Check sheet for the modelled part. Datum: model origin and axes. Units: mm. Face numbers are marked on the shaded views. A direction names the side the tool comes from. Coordinates: 2 decimals unless noted, no trailing zeros. Order: outer loops, then holes, each group sorted by start corner. A loop starts at its lowest first (then second) coordinate and runs counter-clockwise, first axis right, second up. Notation, with made-up numbers: (73.25, 26) -> (110.25, 26) arc R8 ccw to (110.25, 37) -> close; hole circle Ø2 at (88, -24.5). An arc over 180 degrees is marked (long way). Put each result on its own line as item: value. Start each with the question number.
```python
from build123d import *

# Parameters (mm, degrees)
CYLINDER008_R     = 2
CYLINDER008_DEPTH = 3.2
CYLINDER009_R     = 1.7
CYLINDER009_DEPTH = 30
CYLINDER007_R     = 37.75
CYLINDER007_DEPTH = 63
CYLINDER013_R     = 42.75
CYLINDER013_DEPTH = 45
CYLINDER012_R     = 49.75
CYLINDER012_DEPTH = 32.5
SKETCH009_R       = 2.2
POCKET008_DEPTH   = 5
POCKET010_DEPTH   = 25
PAD002_DEPTH      = 5
SKETCH018_W       = 2.5
SKETCH018_H       = 5
POCKET016_DEPTH   = 27.501
SKETCH020_R       = 4
POCKET018_DEPTH   = 5
SKETCH021_R       = 4.4
POCKET019_DEPTH   = 2.5
SKETCH022_R       = 7
POCKET020_DEPTH   = 5
SKETCH023_R       = 1.7
POCKET021_DEPTH   = 5
PAD010_DEPTH      = 15


with BuildPart() as cylinder008:
    # Cylinder008 → Cylinder008 (new body)
    with BuildSketch(Plane.XY.offset(64.8)):
        Circle(CYLINDER008_R)
    extrude(amount=CYLINDER008_DEPTH)


with BuildPart() as fusion005:
    # Cylinder009 → Cylinder009 (new body)
    with BuildSketch(Plane.XY.offset(63)):
        Circle(CYLINDER009_R)
    extrude(amount=CYLINDER009_DEPTH)

    # Fusion005: union Cylinder008
    add(cylinder008.part)


with BuildPart() as cylinder007:
    # Cylinder007 → Cylinder007 (new body)
    with BuildSketch(Plane.XY):
        Circle(CYLINDER007_R)
    extrude(amount=CYLINDER007_DEPTH)


with BuildPart() as fusion006:
    # Cylinder013 → Cylinder013 (new body)
    with BuildSketch(Plane.XY):
        Circle(CYLINDER013_R)
    extrude(amount=CYLINDER013_DEPTH)

    # Fusion006: union Cylinder007
    add(cylinder007.part)


with BuildPart() as obj1:
    # Cylinder012 → Cylinder012 (new body)
    with BuildSketch(Plane.XY.offset(35.5)):
        Circle(CYLINDER012_R)
    extrude(amount=CYLINDER012_DEPTH)

    # Cut008: cut Fusion006
    add(fusion006.part, mode=Mode.SUBTRACT)

    # Cut009: cut Fusion005
    add(fusion005.part, mode=Mode.SUBTRACT)

    # Sketch009 (on Face3 of Cut009) → Pocket008 (cut)
    with BuildSketch(Plane.XY.offset(68)):
        with Locations((0, 28)):
            Circle(SKETCH009_R)
        with Locations((28, 0)):
            Circle(SKETCH009_R)
        with Locations((0, -33)):
            Circle(SKETCH009_R)
        with Locations((-28, 0)):
            Circle(SKETCH009_R)
    extrude(amount=-POCKET008_DEPTH, mode=Mode.SUBTRACT)

    # Sketch011 → Pocket010 (cut)
    with BuildSketch(Plane(origin=(0, 60, -1), x_dir=(1, 0, 0), z_dir=(0, -1, 0))):
        with BuildLine():
            ThreePointArc((3.4, 59.599979), (1.2e-05, 63), (-3.4, 59.600003))
            Line((-3.4, 59.600003), (-3.4, 0))
            Line((-3.4, 0), (3.4, 0))
            Line((3.4, 59.599979), (3.4, 0))
        make_face()
    extrude(amount=POCKET010_DEPTH, mode=Mode.SUBTRACT)

    # Sketch017 (on Face2 of Pocket010) → Pad002 (join)
    with BuildSketch(Plane(origin=(0, 0, 35.5), x_dir=(1, 0, 0), z_dir=(0, 0, -1))):
        with BuildLine():
            ThreePointArc((20.231067, 45.395694), (-0.005277, 49.699749), (-20.240706, 45.391396))
            Line((-7.40759, 82.752427), (-20.240706, 45.391396))
            ThreePointArc((7.358623, 82.756756), (-0.025675, 86.818946), (-7.40759, 82.752427))
            Line((7.358623, 82.756756), (20.231067, 45.395694))
        make_face()
    extrude(amount=-PAD002_DEPTH)

    # Sketch018 (on Face22 of Pad002) → Pocket016 (cut, through all)
    with BuildSketch(Plane(origin=(0, 0, 63), x_dir=(1, 0, 0), z_dir=(0, 0, -1))):
        with Locations((0, 67.5)):
            Rectangle(SKETCH018_W, SKETCH018_H)
    extrude(amount=POCKET016_DEPTH, mode=Mode.SUBTRACT)

    # Sketch020 → Pocket018 (cut)
    with BuildSketch(Plane.XY.offset(68)):
        Circle(SKETCH020_R)
    extrude(amount=-POCKET018_DEPTH, mode=Mode.SUBTRACT)

    # Sketch021 (on Face26 of Pocket018) → Pocket019 (cut)
    with BuildSketch(Plane(origin=(0, 0, 63), x_dir=(1, 0, 0), z_dir=(0, 0, -1))):
        with Locations((0, 33)):
            Circle(SKETCH021_R)
        with Locations((28, 0)):
            Circle(SKETCH021_R)
        with Locations((-28, 0)):
            Circle(SKETCH021_R)
        with Locations((0, -28)):
            Circle(SKETCH021_R)
    extrude(amount=-POCKET019_DEPTH, mode=Mode.SUBTRACT)

    # Sketch022 (on Face2 of Pocket019) → Pocket020 (cut)
    with BuildSketch(Plane.XY.offset(68)):
        Circle(SKETCH022_R)
    extrude(amount=-POCKET020_DEPTH, mode=Mode.SUBTRACT)

    # Sketch023 (on Face2 of Pocket020) → Pocket021 (cut)
    with BuildSketch(Plane.XY.offset(68)):
        with Locations((-15.5, -7)):
            Circle(SKETCH023_R)
        with Locations((15.5, -7)):
            Circle(SKETCH023_R)
        with Locations((-7.75, -20.4)):
            Circle(SKETCH023_R)
        with Locations((7.75, -20.4)):
            Circle(SKETCH023_R)
        with Locations((-7.75, 6.45)):
            Circle(SKETCH023_R)
        with Locations((7.75, 6.45)):
            Circle(SKETCH023_R)
    extrude(amount=-POCKET021_DEPTH, mode=Mode.SUBTRACT)

    # Sketch051 → Pad010 (join)
    with BuildSketch(Plane(origin=(0, 0, 35.5), x_dir=(1, 0, 0), z_dir=(0, 0, -1))):
        with BuildLine():
            Line((3.4, -42), (3.4, -47))
            ThreePointArc((3.4, -47), (0, 47.122818), (-3.4, -47))
            Line((-3.4, -47), (-3.4, -42))
            ThreePointArc((3.4, -42), (0, 42.137394), (-3.4, -42))
        make_face()
    extrude(amount=-PAD010_DEPTH)


with BuildPart() as obj1_1:
    # Body001 placement: moved
    add(obj1.part.moved(Location((0, 0, -68))))


solid = obj1_1.part
```
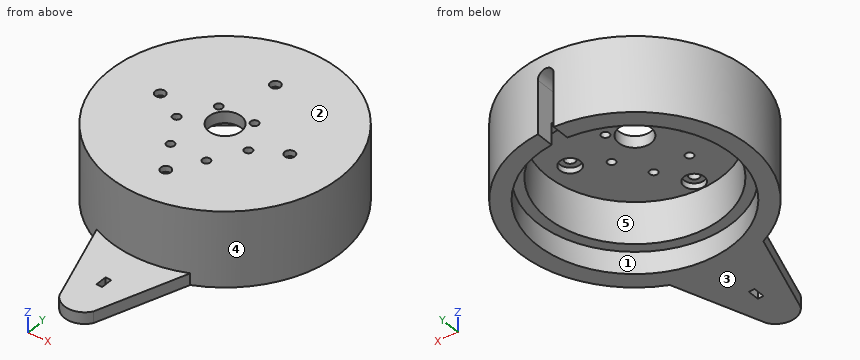
1) Sectioned sample at C-C (x = 15.5). Record the boundary of the cut face in (y, z), plus the area to 3 significant figures.
2) Gauge pin test, flat ends, axial feed: pin 1 (4 mm diameter, centred on x = 7.75, y = -20.4, fed in from -Z); pin 2 (1.5 mm diameter, centred on y = -19.5, z = -6.5, fed in from -X); pin 3 (5 mm diameter, centred on x = 24, z = -18.5, fed in from +Y); pin 4 (7 mm diameter, centred on x = 0, y = 28, fed in from +Z). Record the tip position at first contact, or that the pin passes through.
3) Sectioned sample at D-D (y = -33). Record the boundary of the cut face in (x, z).
4) Sectioned sample at A-A (z = -29.5). Record the boundary of the cut face in (x, y), plus the area to 3 significant figures.
5) Scan lines: line 1 along Y through (x, z) = (0, -1); line 2 along Y through (x, z) = (7.75, -1.1); line 3 along Y through (x, z) = (0, -4). Record each from-to range of solid material in increasing order. Write a range as [from, to].
6) Mould release check, pull along Y, two halves, no side actions. Record for the marked faces 3, 4 and 5: +Y half, -Y half, draft (parallel to the pull), parting line (faces both ways), or undercut.
7) Access from +Z, -Z, +X, -X, +Y, -Y to the whole of each face (thin tool, end or side, straight path). Record for the marked faces 1 and 2.
8) Sectioned sample at B-B (y = 0). State how many separate pieces and enclosed holes the cut face has, plus the area to 3 significant figures.
Entries:
1. outline: (-59.13, -32.5) -> (-39.18, -32.5) -> (-39.18, -23) -> (-34.42, -23) -> (-34.42, -5) -> (-8.7, -5) -> (-8.7, 0) -> (-47.27, 0) -> (-47.27, -27.5) -> (-59.13, -27.5) -> close; (-5.3, -5) -> (34.42, -5) -> (34.42, -23) -> (39.18, -23) -> (39.18, -32.5) -> (47.27, -32.5) -> (47.27, 0) -> (-5.3, 0) -> close
1. area: 1,130 mm2
2. pin 1: stops at z = -5
2. pin 2: stops at x = -46.08
2. pin 3: stops at y = 44.86
2. pin 4: stops at z = 0
3. outline: (-37.23, -32.5) -> (-26.2, -32.5) -> (-26.2, -23) -> (-18.33, -23) -> (-18.33, -5) -> (-4.4, -5) -> (-4.4, -2.5) -> (-2.2, -2.5) -> (-2.2, 0) -> (-37.23, 0) -> close; (2.2, -2.5) -> (4.4, -2.5) -> (4.4, -5) -> (18.33, -5) -> (18.33, -23) -> (26.2, -23) -> (26.2, -32.5) -> (37.23, -32.5) -> (37.23, 0) -> (2.2, 0) -> close
4. outline: (-20.22, -45.46) -> (-7.41, -82.75) arc R8.74 ccw to (7.36, -82.76) -> (20.21, -45.46) arc R49.75 ccw to (3.4, 49.63) -> (3.4, 42) arc R42.14 cw (long way) to (-3.4, 42) -> (-3.4, 49.63) arc R49.75 ccw to start; hole (-1.25, -70) -> (1.25, -70) -> (1.25, -65) -> (-1.25, -65) -> close
4. area: 3,090 mm2
5. line 1: y = [-49.75, -35.2], [-30.8, -7], [7, 25.8], [30.2, 49.75]
5. line 2: y = [-49.14, -22.1], [-18.7, 4.75], [8.15, 49.14]
5. line 3: y = [-49.75, -37.4], [-28.6, -7], [7, 23.6], [32.4, 49.75]
6. face 3: draft
6. face 4: parting line
6. face 5: undercut
7. face 1: -Z
7. face 2: +Z, +X, -X, +Y, -Y
8. separate pieces: 4
8. enclosed holes: 0
8. area: 938 mm2
